Here's how the part is built. I have some questions about the finished solid (model axes, mm). Face numbers are marked on the shaded views. A direction names the side the tool comes from. Coordinates: 2 decimals unless noted, no trailing zeros. Order: outer loops, then holes, each group sorted by start corner. A loop starts at its lowest first (then second) coordinate and runs counter-clockwise, first axis right, second up. Notation, with made-up numbers: (64, 40) - (96, 40) arc R25 cw to (96, 79) - close; hole circle Ø10 at (-28, 17). An arc over 180 degrees is marked (long way). Use one line per item in the form item = value. Start each with the question number.
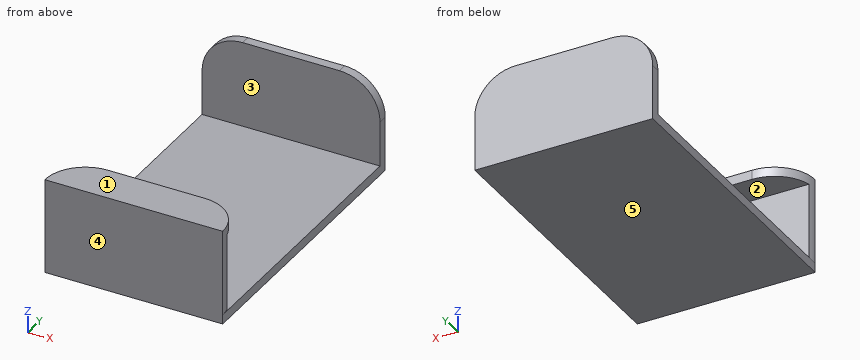
from build123d import *

# Parameters (mm, degrees)
SKETCH2_W               = 57
SKETCH2_H               = 33.5
BOSS_EXTRUDE1_DEPTH     = 100
CUT_EXTRUDE3_DEPTH      = 120.880148482
CUT_EXTRUDE3_DEPTH_BACK = 120.880148482
CUT_EXTRUDE5_DEPTH      = 100
FILLET2_R               = 13


with BuildPart() as part:
    # Sketch2 → Boss-Extrude1 (new body)
    with BuildSketch(Plane(origin=(0, 0, 0), x_dir=(1, 0, 0), z_dir=(0, 1, 0))):
        with Locations((28.5, 16.75)):
            Rectangle(SKETCH2_W, SKETCH2_H)
    extrude(amount=BOSS_EXTRUDE1_DEPTH)

    # Sketch3 → Cut-Extrude3 (cut, two sides: drawn at the far end of the back side and taken through both)
    with BuildSketch(Plane(origin=(57, 0, 0), x_dir=(0, 0, -1), z_dir=(1, 0, 0)).offset(-CUT_EXTRUDE3_DEPTH_BACK)):
        Polygon((0, 100), (0, 97), (30.5, 97), (30.5, 3), (0, 3), (0, 0), (33.5, 0), (33.5, 100), align=None)
    extrude(amount=CUT_EXTRUDE3_DEPTH + CUT_EXTRUDE3_DEPTH_BACK, mode=Mode.SUBTRACT)

    # Sketch4 → Cut-Extrude5 (cut)
    with BuildSketch(Plane(origin=(57, 0, 0), x_dir=(0, 0, -1), z_dir=(1, 0, 0))):
        Polygon((0, 94), (27.5, 94), (27.5, 6), (3, 6), (3, 16), (0, 16), align=None)
    extrude(amount=-CUT_EXTRUDE5_DEPTH, mode=Mode.SUBTRACT)

    # Fillet2
    # the kernel refuses this fillet: 13 mm, written as the material it takes off along each edge
    with BuildSketch(Plane(origin=(0, 61.5, 0), x_dir=(0, 0, -1), z_dir=(0, 1, 0)), Plane(origin=(57, 61.5, 0), x_dir=(-1, 0, 0), z_dir=(0, 1, 0))) as fillet2_piece_1:
        with BuildLine():
            CenterArc((FILLET2_R, -FILLET2_R), FILLET2_R, 90, 90)
            Line((0, -FILLET2_R), (0, 0))
            Line((0, 0), (FILLET2_R, 0))
        make_face()
    extrude(amount=68, mode=Mode.SUBTRACT)
    with BuildSketch(Plane(origin=(57, 16, -35.5), x_dir=(-1, 0, 0), z_dir=(0, 0, 1))) as fillet2_piece_2_section:
        with BuildLine():
            CenterArc((FILLET2_R, FILLET2_R), FILLET2_R, 180, 90)
            Line((0, FILLET2_R), (0, 0))
            Line((0, 0), (FILLET2_R, 0))
        make_face()
    fillet2_piece_2 = extrude(amount=68, mode=Mode.PRIVATE)
    fillet2_piece_2 = split(fillet2_piece_2, bisect_by=Plane(origin=(56.894981294, 5.25203924, -27.5), z_dir=(0, 0, 1)), keep=Keep.TOP, mode=Mode.PRIVATE)
    add(fillet2_piece_2, mode=Mode.SUBTRACT)
    with BuildSketch(Plane(origin=(0, 16, 32.5), x_dir=(0, -1, 0), z_dir=(0, 0, -1))) as fillet2_piece_3_section:
        with BuildLine():
            CenterArc((FILLET2_R, -FILLET2_R), FILLET2_R, 90, 90)
            Line((0, -FILLET2_R), (0, 0))
            Line((0, 0), (FILLET2_R, 0))
        make_face()
    fillet2_piece_3 = extrude(amount=68, mode=Mode.PRIVATE)
    fillet2_piece_3 = split(fillet2_piece_3, bisect_by=Plane(origin=(0.105018706, 5.25203924, -27.5), z_dir=(0, 0, 1)), keep=Keep.TOP, mode=Mode.PRIVATE)
    add(fillet2_piece_3, mode=Mode.SUBTRACT)


solid = part.part
1) Suppose I cut it at A-A, the plane z = -23.5. List the corners of the cut face in (x, y) for me, then the cut area to 3 significant figures.
2) For pin 1 (1.5 mm diameter, centred on x = 16, y = 83.5, fed in from +Z), with a flat end and sliding along its axis, tell me the tip position at first contact or that it passes through.
3) Suppose I cut it at B-B, the plane x = 35.5. List the corners of the cut face in (y, z) for me.
4) If we mould it in two halves opening along Y, with no side actions, what happens to the marked faces 3, 4 and 5? For each: pulls with the +Y half, pulls with the -Y half, needs draft (parallel to the pull), parting line crosses it, or undercut.
5) Suppose I cut it at D-D, the plane y = 24. List the corners of the cut face in (x, z) for me.
6) I need wall thicknesses on probe 1 along Y at (x, z) = (17, -9); probe 2 along Y at (x, z) = (33, -1); probe 3 along Z at (x, y) = (36.5, 8.5). Which ranges of each line are inside material? Lowest first, please. Write a range as [from, to].
7) Which directions (+Z, -Z, +X, -X, +Y, -Y) give clear straight access to the entire face, cutting with the end or side of a thin tool? Please do the marked faces 1 and 2.
8) Suppose I cut it at C-C, the plane z = -4.5. List the corners of the cut face in (x, y) for me, then the cut area to 3 significant figures.
From the geometry:
q1.outline = (0, 3) - (57, 3) arc R13 ccw to (56.65, 6) - (0.35, 6) arc R13 ccw to start; (0, 94) - (57, 94) - (57, 97) - (0, 97) - close
q1.area = 341 mm2
q2.pin_1 = -27.5
q3.outline = (3, -30.5) - (97, -30.5) - (97, 0) - (94, 0) - (94, -27.5) - (6, -27.5) - (6, -3) - (16, -3) - (16, 0) - (3, 0) - close
q4.face_3 = undercut
q4.face_4 = pulls with the -Y half
q4.face_5 = needs draft
q5.outline = (0, -30.5) - (57, -30.5) - (57, -27.5) - (0, -27.5) - close
q6.probe_1 = [3, 6], [94, 97]
q6.probe_2 = [3, 16], [94, 97]
q6.probe_3 = [-30.5, -27.5], [-3, 0]
q7.face_1 = +Z, +X, -X, +Y, -Y
q7.face_2 = +X, -X
q8.outline = (0, 3) - (57, 3) arc R13 ccw to (56.65, 6) - (0.35, 6) arc R13 ccw to start; (3.16, 94) - (53.84, 94) - (53.84, 97) - (3.16, 97) - close
q8.area = 322 mm2
